The model under review builds one solid part; all positions refer to its coordinate system, in mm. Round coordinates to 2 decimals unless told otherwise and drop trailing zeros. Loops run counter-clockwise (first coordinate to the right, second up) from the corner with the lowest first, then second, coordinate; pieces in that order, holes last. Notation, with made-up numbers: (12, 12.5) -> (56, 12.5) arc R27 ccw to (56, 50.5) -> close; hole circle Ø1 at (-1.75, 22). An arc over 180 degrees is marked (long way). Use a Markdown table: item, result. Add a question column.
1) Wall thickness on probe 1 along Z at (x, y) = (457, 2.1); probe 2 along X at (y, z) = (3.9, -154): over which ranges is each line inside the solid? List them lowest first.
2) Consider section B-B on z = -113. Give the boundary of the cut face in (x, y), plus the area to 3 significant figures.
3) Consider section A-A on x = 139. Give the boundary of the cut face in (y, z).
4) Insertion check: pin 1 (2.5 mm diameter, centred on x = 276.5, y = 3.5, fed in from +Z); pin 2 (3 mm diameter, centred on y = 3.5, z = -49.5, fed in from +X); pin 3 (1.5 mm diameter, centred on y = 2, z = -110.5, fed in from -X). Each pin has a flat end and moves straight along its axis. Give the tip position at first contact, or say it passes through.
5) Consider section C-C on y = 3.35. State how many separate pieces and enclosed holes the cut face has, plus the area to 3 significant figures.
from build123d import *

# Parameters (mm, degrees)
CROQUIS1_W              = 64
CROQUIS1_H              = 64
SALIENTE_EXTRUIR1_DEPTH = 5


with BuildPart() as part:
    # Croquis1 → Saliente-Extruir1 (new body)
    with BuildSketch(Plane(origin=(0, 0, 0), x_dir=(1, 0, 0), z_dir=(0, 1, 0))):
        Polygon((-10, -10), (64, -10), (64, -20), (84, -20), (84, -10), (148, -10), (148, -20), (168, -20), (168, -10), (232, -10), (232, -20), (252, -20), (252, -10), (316, -10), (316, -20), (336, -20), (336, -10), (400, -10), (400, -20), (420, -20), (420, -10), (494, -10), (494, 64), (504, 64), (504, 84), (494, 84), (494, 158), (420, 158), (420, 168), (400, 168), (400, 158), (336, 158), (336, 168), (316, 168), (316, 158), (252, 158), (252, 168), (232, 168), (232, 158), (168, 158), (168, 168), (148, 168), (148, 158), (84, 158), (84, 168), (64, 168), (64, 158), (-10, 158), (-10, 84), (-20, 84), (-20, 64), (-10, 64), align=None)
        with Locations((32, 32)):
            Rectangle(CROQUIS1_W, CROQUIS1_H, mode=Mode.SUBTRACT)
        with Locations((116, 32)):
            Rectangle(CROQUIS1_W, CROQUIS1_H, mode=Mode.SUBTRACT)
        with Locations((200, 32)):
            Rectangle(CROQUIS1_W, CROQUIS1_H, mode=Mode.SUBTRACT)
        with Locations((284, 32)):
            Rectangle(CROQUIS1_W, CROQUIS1_H, mode=Mode.SUBTRACT)
        with Locations((368, 32)):
            Rectangle(CROQUIS1_W, CROQUIS1_H, mode=Mode.SUBTRACT)
        with Locations((452, 32)):
            Rectangle(CROQUIS1_W, CROQUIS1_H, mode=Mode.SUBTRACT)
        with Locations((116, 116)):
            Rectangle(CROQUIS1_W, CROQUIS1_H, mode=Mode.SUBTRACT)
        with Locations((200, 116)):
            Rectangle(CROQUIS1_W, CROQUIS1_H, mode=Mode.SUBTRACT)
        with Locations((284, 116)):
            Rectangle(CROQUIS1_W, CROQUIS1_H, mode=Mode.SUBTRACT)
        with Locations((368, 116)):
            Rectangle(CROQUIS1_W, CROQUIS1_H, mode=Mode.SUBTRACT)
        with Locations((452, 116)):
            Rectangle(CROQUIS1_W, CROQUIS1_H, mode=Mode.SUBTRACT)
        with Locations((32, 116)):
            Rectangle(CROQUIS1_W, CROQUIS1_H, mode=Mode.SUBTRACT)
    extrude(amount=SALIENTE_EXTRUIR1_DEPTH)


solid = part.part
Result set:
| question | item | result |
|---|---|---|
| 1 | probe 1 | -158 to -148, -84 to -64, 0 to 10 |
| 1 | probe 2 | -10 to 494 |
| 2 | outline | (-10, 0) -> (0, 0) -> (0, 5) -> (-10, 5) -> close; (64, 0) -> (84, 0) -> (84, 5) -> (64, 5) -> close; (148, 0) -> (168, 0) -> (168, 5) -> (148, 5) -> close; (232, 0) -> (252, 0) -> (252, 5) -> (232, 5) -> close; (316, 0) -> (336, 0) -> (336, 5) -> (316, 5) -> close; (400, 0) -> (420, 0) -> (420, 5) -> (400, 5) -> close; (484, 0) -> (494, 0) -> (494, 5) -> (484, 5) -> close |
| 2 | area | 600 mm2 |
| 3 | outline | (0, -158) -> (5, -158) -> (5, -148) -> (0, -148) -> close; (0, -84) -> (5, -84) -> (5, -64) -> (0, -64) -> close; (0, 0) -> (5, 0) -> (5, 10) -> (0, 10) -> close |
| 4 | pin 1 | z = 10 |
| 4 | pin 2 | x = 494 |
| 4 | pin 3 | x = -10 |
| 5 | separate pieces | 1 |
| 5 | enclosed holes | 12 |
| 5 | area | 37,900 mm2 |
